Model file for the job. Use its own axes, mm. Face numbers are marked on the shaded views. Round coordinates to 2 decimals unless told otherwise and drop trailing zeros. Loops run counter-clockwise (first coordinate to the right, second up) from the corner with the lowest first, then second, coordinate; pieces in that order, holes last. Notation, with made-up numbers: (-37, -23) - (22, -23) arc R17 cw to (22, -6) - close; hole circle Ø8 at (74.5, 37.5). An arc over 180 degrees is marked (long way). Answer as a JSON object with one key per item and string values.
from build123d import *

# Parameters (mm, degrees)
F1_DEPTH      = 63.5
F2_R          = 19.0285497791
F3_DEPTH      = 22.86
F4_R          = 13.812440818
F5_DEPTH      = 0.2070362903
F5_DEPTH_BACK = 61.6676449049


with BuildPart() as f1:
    # F0 (on Top) → F1 (new body)
    with BuildSketch(Plane.XY):
        Polygon((-26.2109767646, -75.7453498801), (56.5097033978, -76.0293745441), (56.5097033978, -37.2225008905), (-26.2109767646, -37.2225008905), align=None)
    extrude(amount=F1_DEPTH)

    # F2 (on face) → F3 (join)
    with BuildSketch(Plane(origin=(-0.2603805333, -75.8344522589, 0), x_dir=(0.9999941055, -0.0034335185, 0), z_dir=(-0.0034335185, -0.9999941055, 0))):
        with Locations((15.1068782434, 32.5047820807)):
            Circle(F2_R)
    extrude(amount=F3_DEPTH)

    # F4 (on face) → F5 (cut, two sides)
    with BuildSketch(Plane(origin=(-0.3388707674, -98.6943175097, 0), x_dir=(0.9999941055, -0.0034335185, 0), z_dir=(-0.0034335185, -0.9999941055, 0))) as f5_sk:
        with Locations((15.1068782434, 32.5047820807)):
            Circle(F4_R)
    extrude(amount=F5_DEPTH, mode=Mode.SUBTRACT)
    extrude(f5_sk.sketch, amount=-F5_DEPTH_BACK, mode=Mode.SUBTRACT)


solid = f1.part
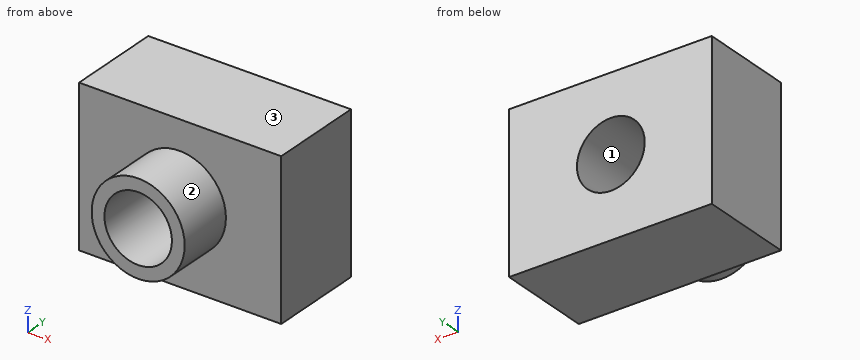
1) Slice it at C-C on x = 46. List the corners of the cut face in (y, z).
Values follow:
{"outline": "(-75.99, 0) - (-37.22, 0) - (-37.22, 63.5) - (-75.99, 63.5) - close"}
2) Drop flat-ended pins along their axis: P1, Ø1.5, axis at y = -91.5, z = 36.5, coming from the +X side; P2, Ø8, axis at y = -82, z = 29.5, coming from the -X side; P3, Ø6, axis at x = 21, z = 11, coming from the -Y side. Give the stop position or say it passes through.
Values follow:
{"P1": "x = 33.54", "P2": "x = -4.21", "P3": "y = -75.92"}
3) Slice it at A-A on z = 33.5. List the corners of the cut face in (x, y).
Values follow:
{"outline": "(-26.21, -75.75) - (-4.16, -75.82) - (-4.23, -98.68) - (0.99, -98.7) - (1.2, -37.22) - (-26.21, -37.22) - close; (28.54, -98.79) - (33.77, -98.81) - (33.85, -75.95) - (56.51, -76.03) - (56.51, -37.22) - (28.76, -37.22) - close"}
4) Slice it at D-D on z = 41.5. List the corners of the cut face in (x, y), then the cut area to 3 significant figures.
Values follow:
{"outline": "(-26.21, -75.75) - (-1.92, -75.83) - (-2, -98.69) - (4.29, -98.71) - (4.5, -37.22) - (-26.21, -37.22) - close; (25.25, -98.78) - (31.54, -98.8) - (31.61, -75.94) - (56.51, -76.03) - (56.51, -37.22) - (25.46, -37.22) - close", "area": "2,680 mm²"}
5) Probe probe 1 along X at (y, z) = (-74, 33.5); probe 2 along Y at (x, z) = (-1, 13.5); probe 3 along Z at (x, y) = (13, -39.5). List the from-to ranges inside material, lowest first.
Values follow:
{"probe 1": "-26.21 to 1.08, 28.63 to 56.51", "probe 2": "-75.83 to -37.22", "probe 3": "0 to 18.83, 46.18 to 63.5"}
6) Slice it at B-B on z = 16. List the corners of the cut face in (x, y), then the cut area to 3 significant figures.
Values follow:
{"outline": "(-26.21, -75.75) - (5.38, -75.85) - (5.3, -98.71) - (24.24, -98.78) - (24.32, -75.92) - (56.51, -76.03) - (56.51, -37.22) - (-26.21, -37.22) - close", "area": "3,630 mm²"}
7) Two-plate mould, pull along Z, no slides. Class the marked faces 1, 2 and 3: pulls with the +Z half, pulls with the -Z half, needs draft (parallel to the pull), parting line crosses it, or undercut.
Values follow:
{"face 1": "undercut", "face 2": "parting line crosses it", "face 3": "pulls with the +Z half"}
